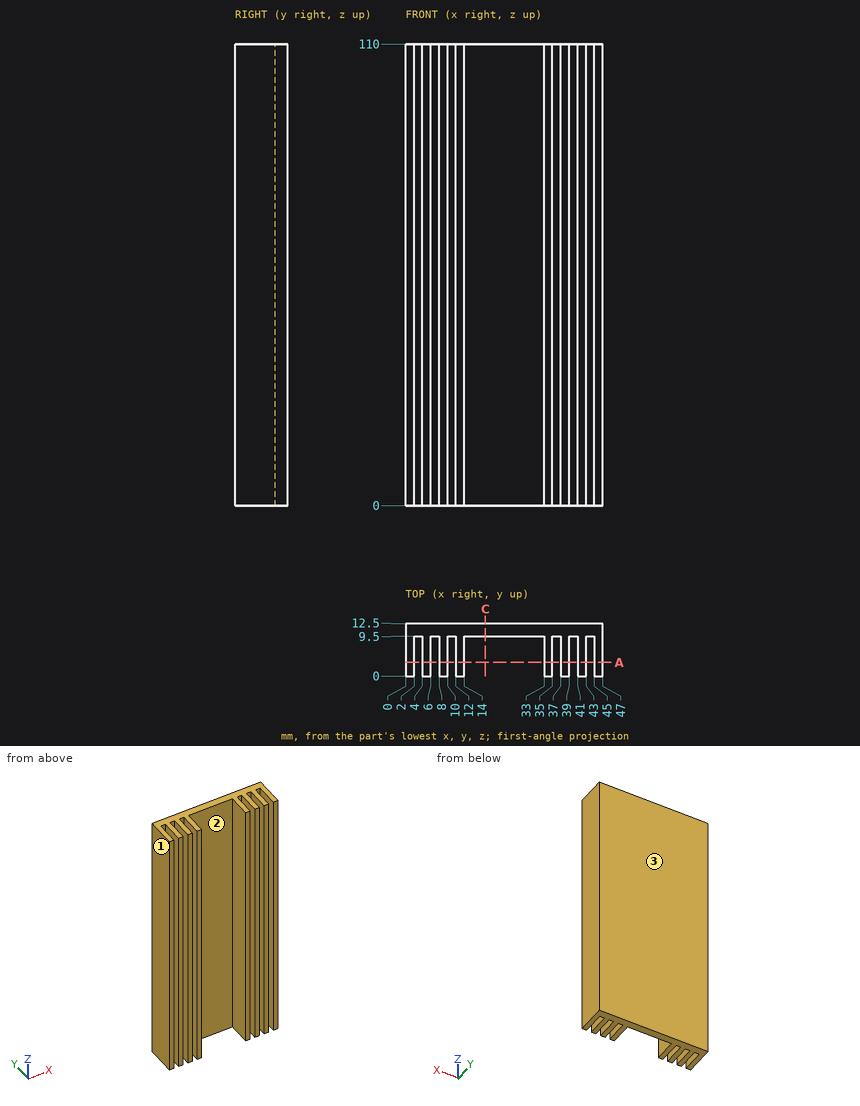
Study the drawing (mm; zero at the part's minimum x, y, z) and answer. Round coordinates to 2 decimals unless told otherwise and drop trailing zeros. Write each loop counter-clockwise with the first axis right and the second up, starting at its lowest first coordinate (ties: lowest second). Pieces come first, ordered by that corner, then holes. Notation, with made-up numbers: (-1, -9.75) - (27, -9.75) arc R28 cw to (27, 10.25) - close; hole circle Ø9 at (56.25, 9). An arc over 180 degrees is marked (long way). Return JSON: item names as keys, results as strings. Group by question number.
Q1. Each of these flat-tipped pins is pushed along its axis until it touches: pin 1 Ø3 at (x, z) = (13.5, 33) entering from -Y; pin 2 Ø1 at (x, z) = (36, 60.5) entering from -Y; pin 3 Ø1.5 at (x, y) = (40, 6) entering from -Z. Where does it stop, or does it pass through?
Q2. Find the intervals of material crossed by L1, parallel to Y at x = 17, z = 78.5, in increasing order.
Q3. The mould has two halves that part along X. Classify the marked faces 1, 2 and 3: released by +X, released by -X, zero draft, split by the parting line, or undercut.
Q4. The part is cut by section C-C on x = 19. Write down the section's boundary in (y, z), then the cut area to 3 significant figures.
Q5. The part is cut by section A-A on y = 3.25. Count the separate pieces of the cut face and the enclosed holes in it, then the cut area to 3 significant figures.
Solved:
{
 "1": {"pin 1": "y = 0", "pin 2": "y = 9.5", "pin 3": "through"},
 "2": {"L1": "9.5 to 12.5"},
 "3": {"face 1": "released by -X", "face 2": "undercut", "face 3": "zero draft"},
 "4": {"outline": "(9.5, 0) - (12.5, 0) - (12.5, 110) - (9.5, 110) - close", "area": "330 mm²"},
 "5": {"separate pieces": "8", "enclosed holes": "0", "area": "1,760 mm²"}
}
